```python
from build123d import *

# Parameters (mm, degrees)
PAD_DEPTH       = 17.5
POCKET_DEPTH    = 12.5
POCKET001_DEPTH = 10
SKETCH003_R     = 1.5
POCKET002_DEPTH = 10
SKETCH004_W     = 10
SKETCH004_H     = 2.5
POCKET003_DEPTH = 41.001
SKETCH010_W     = 4
SKETCH010_H     = 4.25
POCKET008_DEPTH = 12.5
SKETCH011_R     = 1.5
POCKET009_DEPTH = 96.001


with BuildPart() as part:
    # Sketch → Pad (new body)
    with BuildSketch(Plane.XY):
        Polygon((-48, 0), (48, 0), (48, 32.5), (12.5, 32.5), (12.5, 41), (-12.5, 41), (-12.5, 32.5), (-48, 32.5), align=None)
    extrude(amount=PAD_DEPTH)

    # Sketch001 (on Face10 of Pad) → Pocket (cut)
    with BuildSketch(Plane.XY.offset(17.5)):
        Polygon((-48, 27.75), (-43.5, 27.75), (-43.5, 32.5), (-41, 32.5), (-41, 28.25), (-24, 28.25), (-24, 4.25), (-41, 4.25), (-41, 0), (-43.5, 0), (-43.5, 4.75), (-48, 4.75), align=None)
        Polygon((24, 28.25), (41, 28.25), (41, 32.5), (43.5, 32.5), (43.5, 27.75), (48, 27.75), (48, 4.75), (43.5, 4.75), (43.5, 0), (41, 0), (41, 4.25), (24, 4.25), align=None)
    extrude(amount=-POCKET_DEPTH, mode=Mode.SUBTRACT)

    # Sketch002 (on Face8 of Pocket) → Pocket001 (cut)
    with BuildSketch(Plane.XY.offset(17.5)):
        with BuildLine():
            ThreePointArc((-8.5, 31.834849), (-5.428932, 33.928932), (-3.334849, 37))
            Line((-3.334849, 37), (3.334849, 37))
            ThreePointArc((3.334849, 37), (5.428932, 33.928932), (8.5, 31.834849))
            Line((8.5, 31.834849), (8.5, 12.246211))
            ThreePointArc((8.5, 12.246211), (4.732742, 8.865151), (3.334849, 4))
            Line((-3.334849, 4), (3.334849, 4))
            ThreePointArc((-3.334849, 4), (-4.732742, 8.865151), (-8.5, 12.246211))
            Line((-8.5, 31.834849), (-8.5, 12.246211))
        make_face()
    extrude(amount=-POCKET001_DEPTH, mode=Mode.SUBTRACT)

    # Sketch003 (on Face8 of Pocket001) → Pocket002 (cut)
    with BuildSketch(Plane.XY.offset(17.5)):
        with Locations((-8, 36.5)):
            Circle(SKETCH003_R)
        with Locations((8, 36.5)):
            Circle(SKETCH003_R)
        with Locations((-8, 4.5)):
            Circle(SKETCH003_R)
        with Locations((8, 4.5)):
            Circle(SKETCH003_R)
    extrude(amount=-POCKET002_DEPTH, mode=Mode.SUBTRACT)

    # Sketch004 (on Face1 of Pocket002) → Pocket003 (cut, through all)
    with BuildSketch(Plane.XZ):
        with Locations((-20, 1.25)):
            Rectangle(SKETCH004_W, SKETCH004_H)
        with Locations((20, 1.25)):
            Rectangle(SKETCH004_W, SKETCH004_H)
    extrude(amount=-POCKET003_DEPTH, mode=Mode.SUBTRACT)

    # Sketch010 → Pocket008 (cut)
    with BuildSketch(Plane.XY.offset(17.5)):
        with Locations((-30, 30.375)):
            Rectangle(SKETCH010_W, SKETCH010_H)
        with Locations((30, 30.375)):
            Rectangle(SKETCH010_W, SKETCH010_H)
    extrude(amount=-POCKET008_DEPTH, mode=Mode.SUBTRACT)

    # Sketch011 (on Face11 of Pocket008) → Pocket009 (cut, through all)
    with BuildSketch(Plane.YZ.offset(48)):
        with Locations((8.125, 2.5)):
            Circle(SKETCH011_R)
        with Locations((16.25, 2.5)):
            Circle(SKETCH011_R)
        with Locations((24.375, 2.5)):
            Circle(SKETCH011_R)
        with BuildLine():
            ThreePointArc((31.125, 12.25), (30.125, 13.25), (29.125, 12.25))
            Line((29.125, 12.25), (29.125, 10.25))
            ThreePointArc((29.125, 10.25), (30.125, 9.25), (31.125, 10.25))
            Line((31.125, 10.25), (31.125, 12.25))
        make_face()
        with BuildLine():
            ThreePointArc((3.375, 12.25), (2.375, 13.25), (1.375, 12.25))
            Line((1.375, 12.25), (1.375, 10.25))
            ThreePointArc((1.375, 10.25), (2.375, 9.25), (3.375, 10.25))
            Line((3.375, 10.25), (3.375, 12.25))
        make_face()
    extrude(amount=-POCKET009_DEPTH, mode=Mode.SUBTRACT)


solid = part.part
```
Design review of the part built by this model. Coordinates are the model's own, in mm. A direction names the side the tool comes from. Coordinates: 2 decimals unless noted, no trailing zeros. Order: outer loops, then holes, each group sorted by start corner. A loop starts at its lowest first (then second) coordinate and runs counter-clockwise, first axis right, second up. Notation, with made-up numbers: (-18, -25.5) -> (-1, -25.5) arc R19 ccw to (-1, 10.5) -> close; hole circle Ø9 at (62.25, 47). An arc over 180 degrees is marked (long way). One line per item, written item: value. Start each with the question number.
Q1. Insertion check: pin 1 Ø10 at (y, z) = (16, 12.5) entering from -X; pin 2 Ø1.8 at (y, z) = (8.125, 2.5) entering from -X; pin 3 Ø2 at (x, z) = (-46, 11.5) entering from +Y; pin 4 Ø5 at (y, z) = (35.5, 3.5) entering from -X. Each pin has a flat end and moves straight along its axis. Give the tip position at first contact, or say it passes through.
Q2. Take a section at C-C, the plane x = -37. State the section outline as (y, z) points (3 decimals).
Q3. For probe 1 along X at (y, z) = (3.5, 2.25); probe 2 along Y at (x, z) = (-3, 8); probe 3 along Z at (x, y) = (11.5, 16), list the stretches that pass through material, from the lowest coordinate up.
Q4. Tool access review of faces 5 (the flat face through (18, 29.125, 11)), 6 (the flat face through (46, 2, 17.5)), 7 (the flat face through (0, 37, 13)): name each direction out of +Z, -Z, +X, -X, +Y, -Y from which nothing blocks a thin tool from reaching the whole face with its end or side.
Q5. Take a section at A-A, the plane x = -20. State the section outline as (y, z) points (3 decimals).
Q6. Take a section at B-B, the plane y = 16.25. State the section outline as (x, z) points.
Q7. Mouldability with a two-part tool opening along Y and no side actions: class faces 1 (the flat face through (-20, 3, 2.5)), 2 (the cylindrical face through (8, 6, 13)), 3 (the flat face through (-26, 32.5, 9)), 4 (the flat face through (-46, 4.75, 11)) as pulls with the +Y half, pulls with the -Y half, needs draft (parallel to the pull), parting line crosses it, or undercut.
Q8. Take a section at D-D, the plane z = 6.5. Give the number of separate pieces and of enclosed holes in the cut face, then the cut area to 3 significant figures.
Values follow:
1. pin 1: stops at x = -24
1. pin 2: passes through
1. pin 3: stops at y = 32.5
1. pin 4: stops at x = -12.5
2. outline: (0, 0) -> (32.5, 0) -> (32.5, 17.5) -> (28.25, 17.5) -> (28.25, 5) -> (4.25, 5) -> (4.25, 17.5) -> (0, 17.5) -> close; hole (1.375, 10.25) arc R1 ccw to (3.375, 10.25) -> (3.375, 12.25) arc R1 ccw to (1.375, 12.25) -> close; hole circle Ø3 at (8.125, 2.5); hole circle Ø3 at (16.25, 2.5); hole circle Ø3 at (24.375, 2.5); hole (29.125, 10.25) arc R1 ccw to (31.125, 10.25) -> (31.125, 12.25) arc R1 ccw to (29.125, 12.25) -> close
3. probe 1: x = -48 to -25, -15 to 15, 25 to 48
3. probe 2: y = 0 to 4, 37 to 41
3. probe 3: z = 0 to 1.02, 3.98 to 17.5
4. face 5: +X, -X
4. face 6: +Z, +X, -X, +Y, -Y
4. face 7: +Z
5. outline: (0, 2.5) -> (6.625, 2.5) arc R1.5 cw to (9.625, 2.5) -> (14.75, 2.5) arc R1.5 cw to (17.75, 2.5) -> (22.875, 2.5) arc R1.5 cw to (25.875, 2.5) -> (32.5, 2.5) -> (32.5, 17.5) -> (0, 17.5) -> close; hole (1.375, 10.25) arc R1 ccw to (3.375, 10.25) -> (3.375, 12.25) arc R1 ccw to (1.375, 12.25) -> close; hole (29.125, 10.25) arc R1 ccw to (31.125, 10.25) -> (31.125, 12.25) arc R1 ccw to (29.125, 12.25) -> close
6. outline: (-48, 0) -> (-25, 0) -> (-25, 1) -> (-48, 1) -> close; (-48, 4) -> (48, 4) -> (48, 5) -> (24, 5) -> (24, 17.5) -> (8.5, 17.5) -> (8.5, 7.5) -> (-8.5, 7.5) -> (-8.5, 17.5) -> (-24, 17.5) -> (-24, 5) -> (-48, 5) -> close; (-15, 0) -> (15, 0) -> (15, 1) -> (-15, 1) -> close; (25, 0) -> (48, 0) -> (48, 1) -> (25, 1) -> close
7. face 1: needs draft
7. face 2: undercut
7. face 3: pulls with the +Y half
7. face 4: undercut
8. separate pieces: 7
8. enclosed holes: 0
8. area: 2,110 mm2
